```python
from build123d import *

# Parameters (mm, degrees)
ESQUISSE1_W             = 10
ESQUISSE1_H             = 5
BOSS_EXTRU_1_DEPTH      = 110
BOSS_EXTRU_2_DEPTH      = 10
BOSS_EXTRU_3_DEPTH      = 10
ESQUISSE4_W             = 10
ESQUISSE4_H             = 25
BOSS_EXTRU_4_DEPTH      = 10
ESQUISSE5_R             = 2.4
ENL_V_MAT_EXTRU_1_DEPTH = 10
ESQUISSE6_R             = 2.4
ENL_V_MAT_EXTRU_2_DEPTH = 10
CONG_1_R                = 7


with BuildPart() as part:
    # Esquisse1 → Boss.-Extru.1 (new body)
    with BuildSketch(Plane(origin=(0, 0, 0), x_dir=(0, 0, -1), z_dir=(1, 0, 0))):
        Polygon((10, 0), (0, 3.332373658), (0, 0), align=None)
        Polygon((0, 0), (0, -1.93793739), (10, -5.270311049), (10, 0), align=None)
        with Locations((5, -22.5)):
            Rectangle(ESQUISSE1_W, ESQUISSE1_H)
    extrude(amount=BOSS_EXTRU_1_DEPTH)

    # Esquisse2 → Boss.-Extru.2 (add)
    with BuildSketch(Plane.ZY):
        Polygon((0, 3.332373658), (-10, 0), (0, 0), align=None)
        Polygon((0, 0), (-10, 0), (-10, -5.270311049), (0, -1.93793739), align=None)
        Polygon((0, -1.93793739), (-10, -5.270311049), (-10, -25), (0, -25), align=None)
    extrude(amount=BOSS_EXTRU_2_DEPTH)

    # Esquisse3 → Boss.-Extru.3 (add)
    with BuildSketch(Plane(origin=(110, 0, 0), x_dir=(0, 0, -1), z_dir=(1, 0, 0))):
        Polygon((0, 0), (10, 0), (0, 3.332373658), align=None)
        Polygon((10, -5.270311049), (10, 0), (0, 0), (0, -1.93793739), align=None)
        Polygon((10, -25), (10, -5.270311049), (0, -1.93793739), (0, -25), align=None)
    extrude(amount=BOSS_EXTRU_3_DEPTH)

    # Esquisse4 → Boss.-Extru.4 (add)
    with BuildSketch(Plane(origin=(0, 0, -10), x_dir=(-1, 0, 0), z_dir=(0, 0, -1))):
        with Locations((-70, -12.5)):
            Rectangle(ESQUISSE4_W, ESQUISSE4_H)
        with Locations((-40, -12.5)):
            Rectangle(ESQUISSE4_W, ESQUISSE4_H)
    extrude(amount=-BOSS_EXTRU_4_DEPTH)

    # Esquisse5 → Enlèv. mat.-Extru.1 (cut)
    with BuildSketch(Plane(origin=(0, 2.999308969, -0.99948182), x_dir=(1, 0, 0), z_dir=(0, 0.948710608132916, -0.3161458239737997))):
        with Locations(Location((10, 4.216795033, 0), (0, 0, 270))):
            Circle(ESQUISSE5_R)
        with Locations(Location((55, 4.216795033, 0), (0, 0, 270))):
            Circle(ESQUISSE5_R)
        with Locations(Location((100, 4.216795033, 0), (0, 0, 270))):
            Circle(ESQUISSE5_R)
    extrude(amount=-ENL_V_MAT_EXTRU_1_DEPTH, mode=Mode.SUBTRACT)

    # Esquisse6 → Enlèv. mat.-Extru.2 (cut)
    with BuildSketch(Plane.XZ.offset(25)):
        with Locations(Location((10, -5, 0), (0, 0, 270))):
            Circle(ESQUISSE6_R)
        with Locations(Location((55, -5, 0), (0, 0, 270))):
            Circle(ESQUISSE6_R)
        with Locations(Location((100, -5, 0), (0, 0, 270))):
            Circle(ESQUISSE6_R)
    extrude(amount=-ENL_V_MAT_EXTRU_2_DEPTH, mode=Mode.SUBTRACT)

    # Congé1
    cong_1_edges = [part.edges().sort_by_distance(p)[0] for p in [
        (75, -20, -5),
        (65, -20, -5),
        (75, -3.60412422, -5),
        (65, -3.60412422, -5),
        (110, -3.60412422, -5),
        (110, -20, -5),
        (0, -20, -5),
        (0, -3.60412422, -5),
        (35, -20, -5),
        (45, -20, -5),
        (45, -3.60412422, -5),
        (35, -3.60412422, -5),
    ]]
    fillet(cong_1_edges, radius=CONG_1_R)


solid = part.part
```
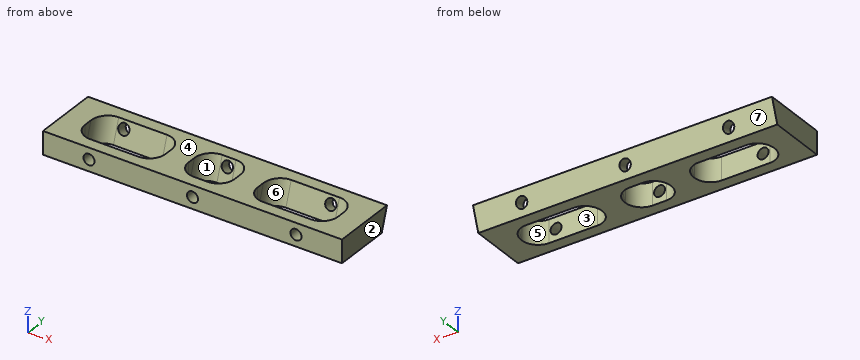
For this review, take the finished solid that the model builds, in its own axes (mm). Face numbers are marked on the shaded views. A direction names the side the tool comes from. Give positions to 0.01 mm unless a question says otherwise; leave off trailing zeros. Order: outer loops, then holes, each group sorted by start corner. A loop starts at its lowest first (then second) coordinate and runs counter-clockwise, first axis right, second up.
1) Insertion check: pin 1 (5 mm diameter, centred on x = 20.5, z = -3.5, fed in from +Y); pin 2 (1.8 mm diameter, centred on x = 56, z = -7.5, fed in from +Y). Each pin has a flat end and moves straight along its axis. Give the tip position at first contact, or say it passes through.
2) Wall thickness on line 1 (X direction, y = -21.6, z = -5); line 2 (X direction, y = -12.75, z = -6.5); line 3 (Y direction, x = 14.5, z = -8): over which ranges is each line inside the solid? List them lowest first.
3) Take a section at A-A (y = -21.75). Give the boundary of the cut face in (x, z).
4) Take a section at D-D (z = -4.25). State how many separate pieces and enclosed holes the cut face has, then the cut area to 3 significant figures.
5) Take a section at B-B (y = -15). Give the boundary of the cut face in (x, z), then the cut area to 3 significant figures.
6) The part is to be moulded in two halves that separate along Y. For the marked faces 4, 5, 6 and 7, say which applies: released by +Y, released by -Y, zero draft, split by the parting line, or undercut.
7) For the marked faces 1, 2 and 3, list the 3-axis set-ups (+Z, -Z, +X, -X, +Y, -Y) from which the entire face can be reached by the end or side of a thin tool; tool diameter is ignored.
8) Take a section at C-C (x = 100). Give the boundary of the cut face in (y, z).
Derived:
1. pin 1: stops at y = 3
1. pin 2: stops at y = 1.08
2. line 1: x = -10 to 7.6, 12.4 to 52.6, 57.4 to 97.6, 102.4 to 120
2. line 2: x = -10 to 0, 35 to 45, 65 to 75, 110 to 120
2. line 3: y = -25 to -20, -4.6 to 0.67
3. outline: (-10, -10) - (120, -10) - (120, 0) - (-10, 0) - close; hole circle Ø4.8 at (10, -5); hole circle Ø4.8 at (55, -5); hole circle Ø4.8 at (100, -5)
4. separate pieces: 4
4. enclosed holes: 0
4. area: 1,990 mm2
5. outline: (-10, -10) - (0.29, -10) - (0.29, 0) - (-10, 0) - close; (34.71, -10) - (45.29, -10) - (45.29, 0) - (34.71, 0) - close; (64.71, -10) - (75.29, -10) - (75.29, 0) - (64.71, 0) - close; (109.71, -10) - (120, -10) - (120, 0) - (109.71, 0) - close
5. area: 418 mm2
6. face 4: zero draft
6. face 5: undercut
6. face 6: undercut
6. face 7: released by +Y
7. face 1: +Z
7. face 2: +Z, -Z, +X, +Y, -Y
7. face 3: +Z, -Z
8. outline: (-25, -10) - (-20, -10) - (-20, -7.4) - (-25, -7.4) - close; (-25, -2.6) - (-20, -2.6) - (-20, 0) - (-25, 0) - close; (-5.27, -10) - (0, -10) - (0.91, -7.28) - (-3.84, -5.7) - close; (-2.32, -1.14) - (2.42, -2.72) - (3.33, 0) - (-1.94, 0) - close
